Input: dimensioned drawing with shaded views. Units: mm. Origin: part minimum x, y, z. A direction names the side the tool comes from. Give positions to 0.01 mm unless a question says otherwise; leave off trailing zeros. Loops run counter-clockwise (first coordinate to the right, second up) from the corner with the lowest first, then second, coordinate; pieces in that order, holes last. Notation, with made-up numbers: M -9,55.5 L 21,55.5 A23 ccw 21,71.5 Z; hole C 69,-21.5 d8. An arc over 180 degrees is marked long. Answer in a Markdown table with one row per item.
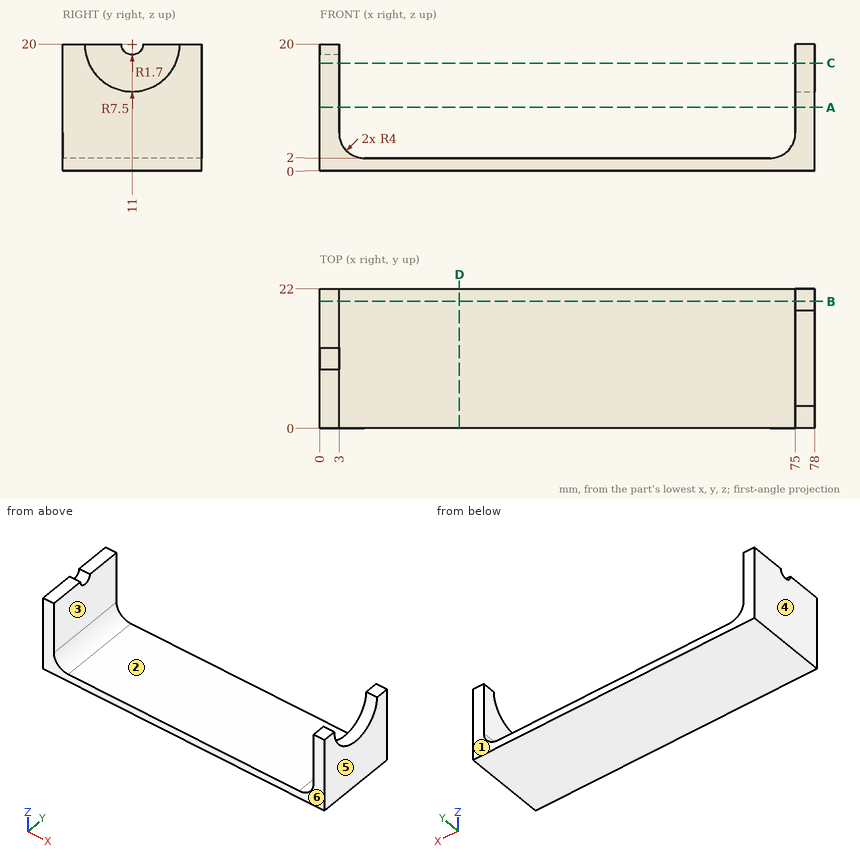
Q1. Ray query, probe 1 along X at (y, z) = (10.25, 8.5); probe 2 along Z at (x, y) = (65.5, 6.5); probe 3 along X at (y, z) = (17.25, 18). Return the intervals inside material, ascending. Write a range as from..to.
Values follow:
| item | result |
|---|---|
| probe 1 | 0..3, 75..78 |
| probe 2 | 0..2 |
| probe 3 | 0..3 |
Q2. Section query A-A (z = 10). Output: boundary loops of the cut face in (x, y), plus the area to 3 significant figures.
Values follow:
| item | result |
|---|---|
| outline | M 0,0 L 3,0 L 3,22 L 0,22 Z; M 75,0 L 78,0 L 78,22 L 75,22 Z |
| area | 132 mm^2 |
Q3. Reachability of the marked faces 1 and 2 from +Z, -Z, +X, -X, +Y, -Y: full face, straight path, thin tool, end or side. Return the list, or none.
Values follow:
| item | result |
|---|---|
| face 1 | +Z, -Z, +X, -X, +Y |
| face 2 | +Z, +Y, -Y |
Q4. Contact query for a flat-ended pin moving along its axis: pin 1 Ø1.5 at (x, y) = (54, 16.5) entering from +Z. Output: stop coordinate, or through.
Values follow:
| item | result |
|---|---|
| pin 1 | z = 2 |
Q5. Section query B-B (y = 20). Output: boundary loops of the cut face in (x, z).
Values follow:
| item | result |
|---|---|
| outline | M 0,0 L 78,0 L 78,20 L 75,20 L 75,6 A4 cw 71,2 L 7,2 A4 cw 3,6 L 3,20 L 0,20 Z |
Q6. Section query D-D (x = 22). Output: boundary loops of the cut face in (y, z).
Values follow:
| item | result |
|---|---|
| outline | M 0,0 L 22,0 L 22,2 L 0,2 Z |
Q7. Section query C-C (z = 17). Output: boundary loops of the cut face in (x, y), plus the area to 3 significant figures.
Values follow:
| item | result |
|---|---|
| outline | M 0,0 L 3,0 L 3,22 L 0,22 Z; M 75,0 L 78,0 L 78,4.13 L 75,4.13 Z; M 75,17.87 L 78,17.87 L 78,22 L 75,22 Z |
| area | 90.8 mm^2 |
Q8. Mould query, pull axis X, two halves, no side actions, for the marked faces 3, 4, 5 and 6. Classes: +X half, -X half, draft (parallel to the pull), parting line (faces both ways), or undercut.
Values follow:
| item | result |
|---|---|
| face 3 | undercut |
| face 4 | -X half |
| face 5 | +X half |
| face 6 | draft |
